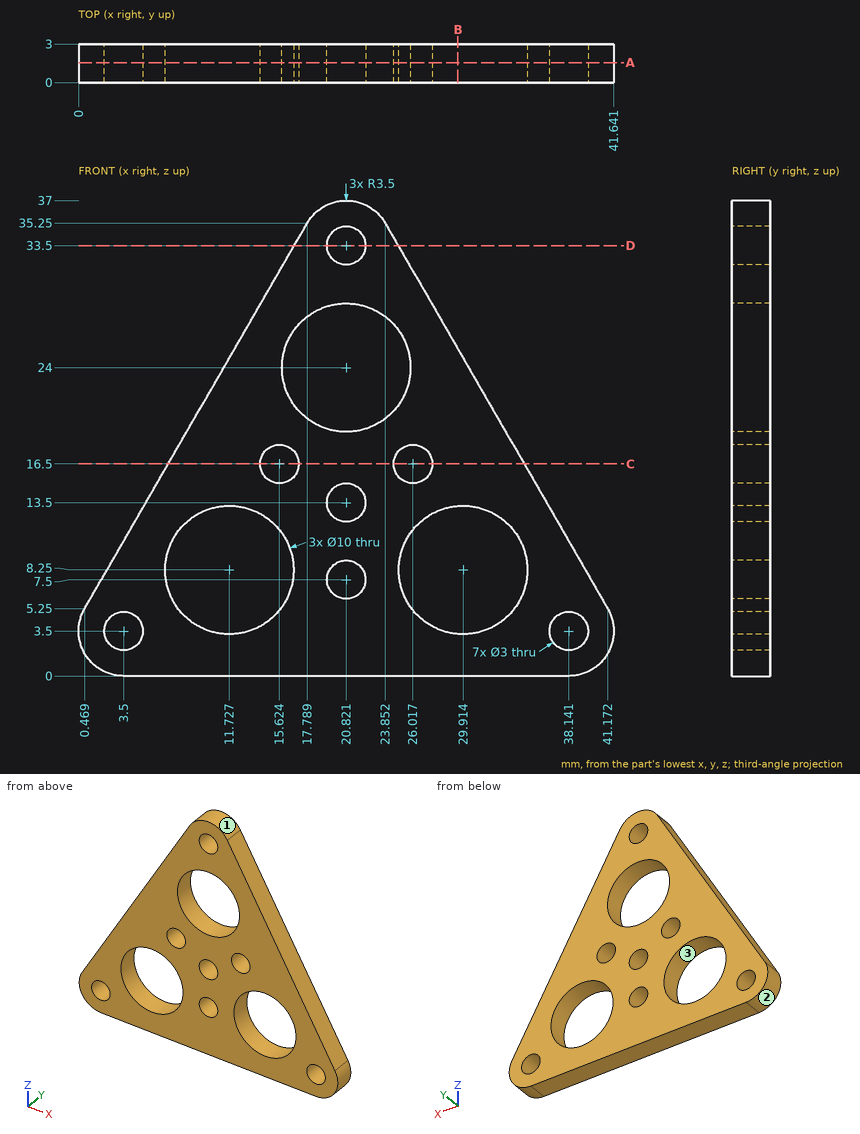
Geometry: see drawing. Coordinates: mm, zero at the bounding-box minimum. Round coordinates to 2 decimals unless told otherwise and drop trailing zeros. Write each loop counter-clockwise with the first axis right and the second up, starting at its lowest first coordinate (ties: lowest second). Pieces come first, ordered by that corner, then holes. Notation, with made-up numbers: M -4.5,9.25 L 47.5,9.25 A22 ccw 47.5,36.25 Z; hole C -22.5,60.5 d8. An arc over 180 degrees is marked long. Answer in a Markdown table with one row per item. Add a question column.
(1) Cut plane C-C, the plane z = 16.5. Return the cut outline in (x, y) (1 decimal).
(2) Cut plane D-D, the plane z = 33.5. Return the cut outline in (x, y).
(3) Cut plane A-A, the plane y = 1.55. Give the number of separate pieces and of enclosed holes in the cut face.
(4) Ray query, L1, parallel to X at y = 1.1, z = 14 (1 decimal); L2, parallel to Z at x = 20, y = 2.3 (1 decimal); L3, parallel to Z at x = 39, y = 2.75 (1 decimal). Return the intervals inside material, ascending.
(5) Cut plane B-B, the plane x = 29.5. Return the cut outline in (y, z).
(6) Contact query for flat-ended pins moving along their axis: pin 1 (3.5 mm diameter, centred on x = 20.82, z = 33.5, fed in from -Y); pin 2 (1 mm diameter, centred on y = 1, z = 6, fed in from +X); pin 3 (8 mm diameter, centred on x = 5.5, z = 23.5, fed in from +Y) (3 decimals). Output: stop coordinate, or through.
(7) Draft query along Z for the marked faces 1, 2 and 3. Return one class per face: pulls with the +Z half, pulls with the -Z half, needs draft (parallel to the pull), parting line crosses it, or undercut.
Established:
| question | item | result |
|---|---|---|
| 1 | outline | M 7,0 L 14.1,0 L 14.1,3 L 7,3 Z; M 17.1,0 L 24.5,0 L 24.5,3 L 17.1,3 Z; M 27.5,0 L 34.7,0 L 34.7,3 L 27.5,3 Z |
| 2 | outline | M 16.78,0 L 19.32,0 L 19.32,3 L 16.78,3 Z; M 22.32,0 L 24.86,0 L 24.86,3 L 22.32,3 Z |
| 3 | separate pieces | 1 |
| 3 | enclosed holes | 10 |
| 4 | L1 | 5.5 to 19.4, 22.2 to 36.1 |
| 4 | L2 | 0 to 6.2, 8.8 to 12.2, 14.8 to 19.1, 28.9 to 32.2, 34.8 to 36.9 |
| 4 | L3 | 0.1 to 2.3, 4.7 to 9 |
| 5 | outline | M 0,0 L 3,0 L 3,3.27 L 0,3.27 Z; M 0,13.23 L 3,13.23 L 3,25.47 L 0,25.47 Z |
| 6 | pin 1 | y = 0 |
| 6 | pin 2 | x = 41.03 |
| 6 | pin 3 | through |
| 7 | face 1 | pulls with the +Z half |
| 7 | face 2 | parting line crosses it |
| 7 | face 3 | undercut |
